from build123d import *

# Parameters (mm, degrees)
SKETCH1_W           = 88
SKETCH1_H           = 93
BOSS_EXTRUDE1_DEPTH = 13
CUT_EXTRUDE1_DEPTH  = 11.5
CUT_EXTRUDE2_DEPTH  = 66.324191537
BOSS_EXTRUDE2_DEPTH = 7.5


with BuildPart() as part:
    # Sketch1 → Boss-Extrude1 (new body)
    with BuildSketch(Plane(origin=(0, 0, 0), x_dir=(1, 0, 0), z_dir=(0, 1, 0))):
        Rectangle(SKETCH1_W, SKETCH1_H)
    extrude(amount=BOSS_EXTRUDE1_DEPTH)

    # Sketch2 → Cut-Extrude1 (cut)
    with BuildSketch(Plane(origin=(0, 13, 0), x_dir=(1, 0, 0), z_dir=(0, 1, 0))):
        Polygon((-44, -36.5), (-44, -46.5), (-34, -46.5), (34, -46.5), (44, -46.5), (44, -36.5), (44, 36.5), (44, 46.5), (34, 46.5), (-34, 46.5), (-44, 46.5), (-44, 36.5), align=None)
        Polygon((-30, -43), (-40.5, -32.5), (-40.5, 32.5), (-30, 43), (30, 43), (40.5, 32.5), (40.5, -32.5), (30, -43), align=None, mode=Mode.SUBTRACT)
    extrude(amount=-CUT_EXTRUDE1_DEPTH, mode=Mode.SUBTRACT)

    # Sketch3 → Cut-Extrude2 (cut, through all)
    with BuildSketch(Plane(origin=(0, 13, 0), x_dir=(1, 0, 0), z_dir=(0, 1, 0))):
        Polygon((-29.378679656, -41.5), (29.378679656, -41.5), (39, -31.878679656), (39, 31.878679656), (29.378679656, 41.5), (-29.378679656, 41.5), (-39, 31.878679656), (-39, -31.878679656), align=None)
    extrude(amount=-CUT_EXTRUDE2_DEPTH, mode=Mode.SUBTRACT)

    # Sketch5 → Boss-Extrude2 (add)
    with BuildSketch(Plane(origin=(-39, 0, 0), x_dir=(0, 0, -1), z_dir=(1, 0, 0))):
        with BuildLine():
            Line((-6.25, 0), (6.25, 0))
            Line((6.25, 0), (6.25, 8))
            Line((6.25, 8), (3.25, 8))
            ThreePointArc((3.25, 8), (0, 4.75), (-3.25, 8))
            Line((-3.25, 8), (-6.25, 8))
            Line((-6.25, 8), (-6.25, 0))
        make_face()
    boss_extrude2 = extrude(amount=BOSS_EXTRUDE2_DEPTH)

    # Mirror1: Boss-Extrude2 across plane
    add(boss_extrude2.mirror(Plane(origin=(0, 0, 0), x_dir=(0, 0, 1), z_dir=(1, 0, 0))))


solid = part.part
Part model, mm, in its own coordinate system. A direction names the side the tool comes from. Give positions to 0.01 mm unless a question says otherwise; leave off trailing zeros. Loops run counter-clockwise (first coordinate to the right, second up) from the corner with the lowest first, then second, coordinate; pieces in that order, holes last.
(1) Drill centre lines: line 1 along Z through (x, y) = (-13, 1); line 2 along Z through (x, y) = (29, 11.25); line 3 along X through (y, z) = (3.5, -10). Where is each one in solid material? Low to high.
Return value:
line 1: z = -46.5 to -41.5, 41.5 to 46.5
line 2: z = -43 to -41.5, 41.5 to 43
line 3: x = -40.5 to -39, 39 to 40.5
(2) Band-saw the part on D-D (z = 0). Write the cut outline in (x, y), and give its area (3 significant figures).
Return value:
outline: (-44, 0) - (-31.5, 0) - (-31.5, 4.75) - (-39, 4.75) - (-39, 13) - (-40.5, 13) - (-40.5, 1.5) - (-44, 1.5) - close; (31.5, 0) - (44, 0) - (44, 1.5) - (40.5, 1.5) - (40.5, 13) - (39, 13) - (39, 4.75) - (31.5, 4.75) - close
area: 121 mm2
(3) Band-saw the part on C-C (y = 11.5). Write the cut outline in (x, z), and give its area (3 significant figures).
Return value:
outline: (-40.5, -32.5) - (-30, -43) - (30, -43) - (40.5, -32.5) - (40.5, 32.5) - (30, 43) - (-30, 43) - (-40.5, 32.5) - close; hole (-39, -31.88) - (-29.38, -41.5) - (29.38, -41.5) - (39, -31.88) - (39, 31.88) - (29.38, 41.5) - (-29.38, 41.5) - (-39, 31.88) - close
area: 457 mm2
(4) Pull direction X, two halves, no side cores. Call faces 1 (the flat face through (-40.5, 7, 0)), 2 (the cylindrical face through (35.3, 4.75, -0.07)), 3 (the flat face through (-3, 1.5, 45)): pulls with the +X half, pulls with the -X half, needs draft (parallel to the pull), parting line crosses it, or undercut.
Return value:
face 1: pulls with the -X half
face 2: undercut
face 3: needs draft
(5) Band-saw the part on A-A (z = -11.5). Write the cut outline in (x, y).
Return value:
outline: (-44, 0) - (-39, 0) - (-39, 13) - (-40.5, 13) - (-40.5, 1.5) - (-44, 1.5) - close; (39, 0) - (44, 0) - (44, 1.5) - (40.5, 1.5) - (40.5, 13) - (39, 13) - close
(6) 3-axis set-ups, long thin cutter, end or side, ignore diameter. For faces 4 (the flat face through (0, 7, 41.5)), 5 (the flat face through (-33, 0, -4)), 6 (the flat face through (35, 8, 5)), 7 (the flat face through (-35, 7, -38)): which of +Z, -Z, +X, -X, +Y, -Y reach the whole face in a straight line?
Return value:
face 4: +Y, -Y
face 5: +Z, -Z, +X, -X, -Y
face 6: +Y
face 7: -Z, -X, +Y
(7) Band-saw the part on B-B (x = 28). Write the cut outline in (y, z), and give its area (3 significant figures).
Return value:
outline: (0, -46.5) - (1.5, -46.5) - (1.5, -43) - (13, -43) - (13, -41.5) - (0, -41.5) - close; (0, 41.5) - (13, 41.5) - (13, 43) - (1.5, 43) - (1.5, 46.5) - (0, 46.5) - close
area: 49.5 mm2
(8) Pin check, flat tips, straight feed: pin 1 (5 mm diameter, centred on x = -1.5, y = 10.5, fed in from -Z); pin 2 (6 mm diameter, centred on y = 8, z = -36.5, fed in from +X); pin 3 (6.5 mm diameter, centred on y = 3.5, z = -0.5, fed in from -X); pin 4 (2 mm diameter, centred on x = -37, y = 5, fed in from +Z). Stop position of each tip, or through.
Return value:
pin 1: stops at z = -43
pin 2: stops at x = 39.5
pin 3: stops at x = -44
pin 4: stops at z = 37
